Geometry: final body of the model. Coordinates: model frame, mm. Face numbers are marked on the shaded views. A direction names the side the tool comes from. Coordinates: 2 decimals unless noted, no trailing zeros. Order: outer loops, then holes, each group sorted by start corner. A loop starts at its lowest first (then second) coordinate and runs counter-clockwise, first axis right, second up. Notation, with made-up numbers: (14.5, 58.5) -> (29.5, 58.5) arc R7 ccw to (29.5, 63.5) -> close; hole circle Ø10 at (-7, 0). An arc over 180 degrees is marked (long way). Use one line per item in the form item = value.
```python
from build123d import *

# Parameters (mm, degrees)
F0_R     = 5.842
F1_DEPTH = 17.78
F3_DEPTH = 15.24
F4_R     = 6.985
F4_R_2   = 5.842
F5_DEPTH = 2.54


# Not quite as in the source:
# - a fillet or chamfer that OpenCascade refuses, or shapes differently, is made with other operations: its cross-section is extruded or revolved along the edge and cut away or added


with BuildPart() as f1:
    # F0 (on Top) → F1 (new body)
    with BuildSketch(Plane.XY):
        Circle(F0_R)
    extrude(amount=F1_DEPTH)

    # F2 (on face) → F3 (cut)
    with BuildSketch(Plane.XY.offset(17.78)):
        with BuildLine():
            Line((1.27, -5.7022858574), (1.27, 5.7022858574))
            ThreePointArc((1.27, 5.7022858574), (0, 5.842), (-1.27, 5.7022858574))
            Line((-1.27, 5.7022858574), (-1.27, -5.7022858574))
            ThreePointArc((-1.27, -5.7022858574), (0, -5.842), (1.27, -5.7022858574))
        make_face()
    extrude(amount=-F3_DEPTH, mode=Mode.SUBTRACT)

    # F4 (on face) → F5 (join)
    with BuildSketch(Plane(origin=(0, 0, 0), x_dir=(1, 0, 0), z_dir=(0, 0, -1))):
        Circle(F4_R)
        Circle(F4_R_2, mode=Mode.SUBTRACT)
        Circle(F4_R_2)
    extrude(amount=F5_DEPTH)

    # F6: fillet of radius 5.08 on 1 edges, made by hand

    # F6_s1 → F6_t2 (revolve, cut)
    with BuildSketch(Plane.XZ):
        with BuildLine():
            ThreePointArc((6.985, 0), (5.1255909488, -1.8594090512), (2.5855909488, -2.54))
            Line((2.5855909488, -2.54), (6.985, -2.54))
            Line((6.985, -2.54), (6.985, 0))
        make_face()
    revolve(axis=Axis((0, 0, -2.54), (0, 0, -1)), mode=Mode.SUBTRACT)


solid = f1.part
```
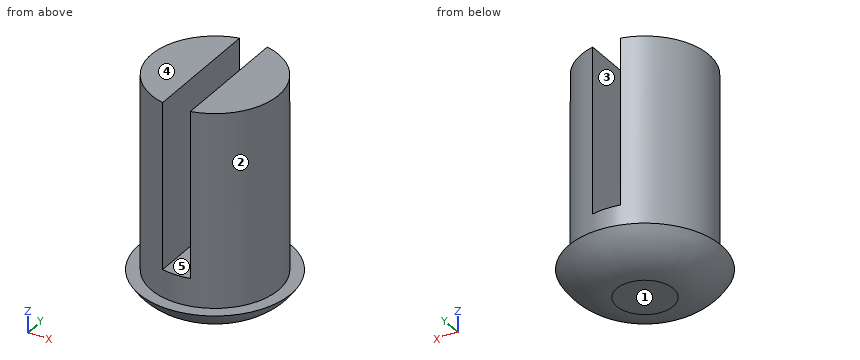
1) Access query for the marked faces 4 and 5. Directions: +Z, -Z, +X, -X, +Y, -Y. A direction counts if a zero-diameter tool reaches every point of the face in a straight line with its end or side. Return the directions, or none.
Results found:
face_4 = +Z, +X, -X, +Y, -Y
face_5 = +Z, +Y, -Y
2) Contact query for flat-ended pins moving along their axis: P1, Ø6, axis at y = -4, z = 5, coming from the -X side; P2, Ø3, axis at x = 0.5, y = 2.5, coming from the +Z side; P3, Ø2, axis at x = 0, z = 13.5, coming from the +Y side; P4, Ø3, axis at y = -3, z = 3, coming from the +X side. Output: stop coordinate, or through.
Results found:
P1 = -5.76
P2 = 17.78
P3 = through
P4 = 5.65
3) Section B-B, the plane z = 0.75. Output: boundary loops of the cut face in (x, y).
Results found:
outline = circle Ø11.68 at (0, 0)
4) Section A-A, the plane z = 3.5. Output: boundary loops of the cut face in (x, y).
Results found:
outline = (-1.27, -5.7) -> (-1.27, 5.7) arc R5.84 ccw to start; (1.27, -5.7) arc R5.84 ccw to (1.27, 5.7) -> close
5) Material intervals for probe 1 along X at (y, z) = (-0.25, 4.5); probe 2 along X at (y, z) = (-1.25, 6); probe 3 along Y at (x, z) = (0, 0.5), sorted ascending. Write a range as from..to.
Results found:
probe_1 = -5.84..-1.27, 1.27..5.84
probe_2 = -5.71..-1.27, 1.27..5.71
probe_3 = -5.84..5.84
6) Pull-direction query (X, two-part tool) for the marked faces 1, 2 and 3; classes: released by +X, released by -X, zero draft, split by the parting line, or undercut.
Results found:
face_1 = zero draft
face_2 = split by the parting line
face_3 = undercut
